from build123d import *

# Parameters (mm, degrees)
SKETCH1_W           = 70
SKETCH1_H           = 29
SKETCH1_R           = 1.5
BOSS_EXTRUDE1_DEPTH = 2
SKETCH3_W           = 39.225392784
SKETCH3_H           = 21.196798794
BOSS_EXTRUDE2_DEPTH = 7
FILLET2_R           = 7
FILLET3_R           = 7


with BuildPart() as part:
    # Sketch1 → Boss-Extrude1 (new body)
    with BuildSketch(Plane(origin=(0, 0, 0), x_dir=(1, 0, 0), z_dir=(0, 1, 0))):
        Rectangle(SKETCH1_W, SKETCH1_H)
        with Locations(Location((-30.499583195, 10.498163925, 0), (0, 0, 270))):
            Circle(SKETCH1_R, mode=Mode.SUBTRACT)
        with Locations(Location((30.500416805, 10.498163925, 0), (0, 0, 270))):
            Circle(SKETCH1_R, mode=Mode.SUBTRACT)
        with Locations(Location((-30.499583195, -10.501836075, 0), (0, 0, 270))):
            Circle(SKETCH1_R, mode=Mode.SUBTRACT)
        with Locations(Location((30.500416805, -10.501836075, 0), (0, 0, 270))):
            Circle(SKETCH1_R, mode=Mode.SUBTRACT)
    extrude(amount=BOSS_EXTRUDE1_DEPTH)

    # Sketch3 → Boss-Extrude2 (add)
    with BuildSketch(Plane(origin=(0, 2, 0), x_dir=(1, 0, 0), z_dir=(0, 1, 0))):
        Rectangle(SKETCH3_W, SKETCH3_H)
    extrude(amount=BOSS_EXTRUDE2_DEPTH)

    # Fillet2
    # the kernel refuses this fillet: 7 mm, written as the material it adds along each edge
    with BuildSketch(Plane(origin=(-19.612696392, 2, 10.598399397), x_dir=(0, 0, 1), z_dir=(1, 0, 0)), Plane(origin=(19.612696392, 2, -10.598399397), x_dir=(0, 0, -1), z_dir=(-1, 0, 0))) as fillet2_piece_1:
        with BuildLine():
            CenterArc((7, -6.276935652), FILLET2_R, 116.271709478, 63.728290522)
            Line((0, -6.276935652), (-0.14, -6.276935652))
            Line((-0.14, -6.276935652), (-0.14, 0))
            Line((-0.14, 0), (0, 0.14))
            ThreePointArc((0, 0.14), (1.950800302, 0.14), (3.839632616, 0.125538713))
            Line((3.839632616, 0.125538713), (3.901600603, 0))
        make_face()
    extrude(amount=39.225392784)

    # Fillet3
    fillet3_edges = [part.edges().sort_by_distance(p)[0] for p in [
        (0, 9, -10.598399397),
        (0, 9, 10.598399397),
    ]]
    fillet(fillet3_edges, radius=FILLET3_R)


solid = part.part
Geometry check sheet. Reference: the model listing, model coordinates, mm. A direction names the side the tool comes from. Round coordinates to 2 decimals unless told otherwise and drop trailing zeros. Order: outer loops, then holes, each group sorted by start corner. A loop starts at its lowest first (then second) coordinate and runs counter-clockwise, first axis right, second up. Notation, with made-up numbers: (76.25, 9) -> (116.25, 9) arc R27 ccw to (116.25, 30) -> close; hole circle Ø4 at (51.25, 51.25). An arc over 180 degrees is marked (long way). Use one line per item in the form item = value.
1. Cross-section at A-A, the plane z = -4. Enter the section's corners in (x, y), plus the area to 3 significant figures.
Working result:
outline = (-35, 0) -> (35, 0) -> (35, 2) -> (19.61, 2) -> (19.61, 9) -> (-19.61, 9) -> (-19.61, 2) -> (-35, 2) -> close
area = 415 mm^2
2. Scan lines: line 1 along X through (y, z) = (3.25, 1); line 2 along Z through (x, y) = (-31, 1.5); line 3 along Y through (x, z) = (30, -3.75). Record each from-to range of solid material in increasing order. Write a range as from..to.
Working result:
line_1 = -19.61..19.61
line_2 = -14.5..-11.91, -9.08..9.09, 11.92..14.5
line_3 = 0..2
3. Cross-section at C-C, the plane z = 9.75. Count the separate pieces of the cut face and the enclosed holes in it, plus the area to 3 significant figures.
Working result:
separate_pieces = 3
enclosed_holes = 0
area = 334 mm^2
4. Cross-section at B-B, the plane x = -22.5. Enter the section's corners in (y, z), plus the area to 3 significant figures.
Working result:
outline = (0, -14.5) -> (2, -14.5) -> (2, 14.5) -> (0, 14.5) -> close
area = 58.0 mm^2
5. Set-up check for faces 5 (the face through (27, 2, 0)), 6 (the face through (0, 3, 13)), 7 (the face through (-27, 2, 0)): record each of +Z, -Z, +X, -X, +Y, -Y from which the full face is reachable in a straight line by a thin tool's end or side.
Working result:
face_5 = +Z, -Z, +X, +Y
face_6 = +Z, +X, -X, +Y
face_7 = +Z, -Z, -X, +Y
6. Mould release check, pull along X, two halves, no side actions. Record for faces 1 (the face through (0, 0, 0)), 2 (the face through (35, 1, 0)), 3 (the face through (-19.613, 5, 0)), 4 (the face through (-29.235, 0.986, -9.692)): pulls with the +X half, pulls with the -X half, needs draft (parallel to the pull), parting line crosses it, or undercut.
Working result:
face_1 = needs draft
face_2 = pulls with the +X half
face_3 = pulls with the -X half
face_4 = undercut
7. Go/stop test with flat-tipped pins: pin 1 (17 mm diameter, centred on x = 29.5, z = 6.5, fed in from +Y); pin 2 (2.5 mm diameter, centred on x = -30.5, z = -10.5, fed in from +Y); pin 3 (2 mm diameter, centred on y = 5, z = -3, fed in from +X); pin 4 (2 mm diameter, centred on y = 6, z = -1, fed in from -X). Record where each tip stops, or that it passes through.
Working result:
pin_1 = 2
pin_2 = through
pin_3 = 19.61
pin_4 = -19.61
